For this review, take the finished solid that the model builds, in its own axes (mm). Face numbers are marked on the shaded views. A direction names the side the tool comes from. Round coordinates to 2 decimals unless told otherwise and drop trailing zeros. Write each loop counter-clockwise with the first axis right and the second up, starting at its lowest first coordinate (ties: lowest second). Pieces come first, ordered by that corner, then holes. Notation, with made-up numbers: M 32.5,-32 L 66.5,-32 A18 ccw 66.5,-14 Z; hole C 40,21 d8. An arc over 180 degrees is marked long. Use one line per item in the form item = value. Start each with the question number.
Item 1: Add section D-D (z = -26). State the section outline as (x, y) points, and give its area (3 significant figures).
Item 2: For the marked faces 1, 2 and 3, list the 3-axis set-ups (+Z, -Z, +X, -X, +Y, -Y) from which the entire face can be reached by the end or side of a thin tool; tool diameter is ignored.
Item 3: For line 1 (X direction, y = 2.5, z = -29); line 2 (X direction, y = 3.75, z = -4.5); line 3 (Z direction, x = 15, y = 2.75), list the stretches that pass through material, from the lowest coordinate up. Write a range as [from, to].
Item 4: Add section C-C (x = 35). State the section outline as (y, z) points.
Item 5: For P1, Ø16, axis at x = 29, z = -17.5, coming from the +Y side; P2, Ø4, axis at x = 36, y = 7.5, coming from the -Z side; P3, Ø1.5, axis at y = 3, z = -20.5, coming from the +X side; P4, Ø2, axis at y = 3.5, z = -26.5, coming from the +X side, all flat-tipped, find the tip position at first contact; note any pin that passes through.
Item 6: Add section B-B (z = -13). State the section outline as (x, y) points.
Item 7: Add section A-A (y = 3). State the section outline as (x, z) points.
Item 8: Draft analysis for pull direction X (two halves, no side actions). For the marked faces 4, 5 and 6, state which applies: released by +X, released by -X, zero draft, split by the parting line, or undercut.
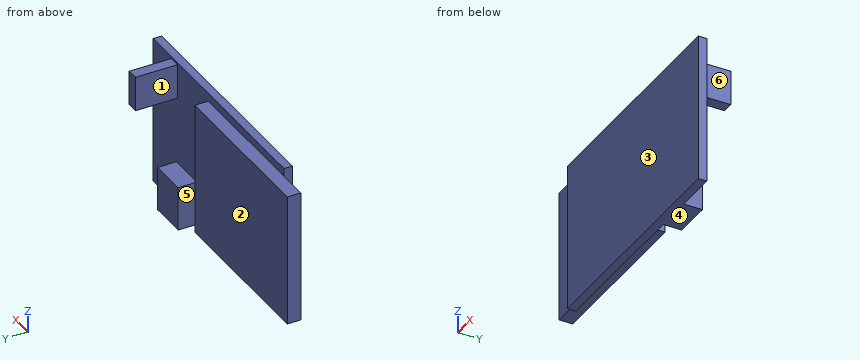
from build123d import *

# Parameters (mm, degrees)
SKETCH1_W           = 51
SKETCH1_H           = 32
BOSS_EXTRUDE1_DEPTH = 1.8
SKETCH2_W           = 36
SKETCH2_H           = 28.5
BOSS_EXTRUDE2_DEPTH = 2.9
SKETCH3_W           = 2.4
SKETCH3_H           = 7.5
BOSS_EXTRUDE3_DEPTH = 9
SKETCH4_W           = 8
SKETCH4_H           = 9.5
BOSS_EXTRUDE4_DEPTH = 4


with BuildPart() as part:
    # Sketch1 → Boss-Extrude1 (new body)
    with BuildSketch(Plane(origin=(0, 0, 0), x_dir=(1, 0, 0), z_dir=(0, 1, 0))):
        with Locations((25.5, 16)):
            Rectangle(SKETCH1_W, SKETCH1_H)
    extrude(amount=BOSS_EXTRUDE1_DEPTH)

    # Sketch2 → Boss-Extrude2 (add)
    with BuildSketch(Plane(origin=(0, 1.8, 0), x_dir=(1, 0, 0), z_dir=(0, 1, 0))):
        with Locations((11.5, 16)):
            Rectangle(SKETCH2_W, SKETCH2_H)
    extrude(amount=BOSS_EXTRUDE2_DEPTH)

    # Sketch3 → Boss-Extrude3 (add)
    with BuildSketch(Plane(origin=(0, 1.8, 0), x_dir=(1, 0, 0), z_dir=(0, 1, 0))):
        with Locations((42.8, 4.25)):
            Rectangle(SKETCH3_W, SKETCH3_H)
    extrude(amount=BOSS_EXTRUDE3_DEPTH)

    # Sketch4 → Boss-Extrude4 (add)
    with BuildSketch(Plane(origin=(0, 1.8, 0), x_dir=(1, 0, 0), z_dir=(0, 1, 0))):
        with Locations((38, 27.25)):
            Rectangle(SKETCH4_W, SKETCH4_H)
    extrude(amount=BOSS_EXTRUDE4_DEPTH)


solid = part.part
Calculated:
q1.outline = M -6.5,1.8 L 0,1.8 L 0,0 L 51,0 L 51,1.8 L 42,1.8 L 42,5.8 L 34,5.8 L 34,1.8 L 29.5,1.8 L 29.5,4.7 L -6.5,4.7 Z
q1.area = 228 mm^2
q2.face_1 = +Z, +Y
q2.face_2 = +Z, -Z, -X, +Y
q2.face_3 = +Z, -Z, +X, -X, -Y
q3.line_1 = [-6.5, 29.5], [34, 42]
q3.line_2 = [-6.5, 29.5], [41.6, 44]
q3.line_3 = [-30.25, -1.75]
q4.outline = M 0,-32 L 5.8,-32 L 5.8,-22.5 L 1.8,-22.5 L 1.8,0 L 0,0 Z
q5.P1 = 5.8
q5.P2 = -32
q5.P3 = 29.5
q5.P4 = 42
q6.outline = M -6.5,1.8 L 0,1.8 L 0,0 L 51,0 L 51,1.8 L 29.5,1.8 L 29.5,4.7 L -6.5,4.7 Z
q7.outline = M -6.5,-30.25 L 29.5,-30.25 L 29.5,-1.75 L -6.5,-1.75 Z; M 34,-32 L 42,-32 L 42,-22.5 L 34,-22.5 Z; M 41.6,-8 L 44,-8 L 44,-0.5 L 41.6,-0.5 Z
q8.face_4 = zero draft
q8.face_5 = undercut
q8.face_6 = released by +X
